Read the model definition and answer for the solid it produces. Units are mm, in the model's axes. A direction names the side the tool comes from. Coordinates: 2 decimals unless noted, no trailing zeros. Write each loop counter-clockwise with the first axis right and the second up, starting at its lowest first coordinate (ties: lowest second). Pieces come first, ordered by that corner, then holes.
(1) Which of the six approach directions +Z, -Z, +X, -X, +Y, -Y give full straight-line access (tool end or side, diameter ignored) to faces 4 (the cylindrical face through (-20.03, 6.31, 1.48)), 5 (the flat face through (-3, 14, 30)), 6 (the flat face through (-1, 16, 5))?
(2) Given pin 1 (21.5 mm diameter, centred on x = -9, y = -5, fed in from -Z); pin 2 (8 mm diameter, centred on y = 8, z = 17, fed in from +X); pin 3 (3 mm diameter, centred on x = 1, z = 19, fed in from -Y); pin 4 (12 mm diameter, centred on x = 14.5, z = 8.5, fed in from -Y), each flat-ended and moving along its own axis, determine where each tip first touches the part or whether it passes through.
(3) The part is cut by section A-A, the plane y = 0. Determine the outline of the cut face in (x, z).
(4) Straight lines are drawn through the part: line 1 along X through (y, z) = (0, 11); line 2 along Z through (x, y) = (16, 5.5). For each, find the intervals that lie inside material, in ascending order.
(5) Determine the mould class of faces 1 (the cylindrical face through (-12.932, -5.362, 14.79)), 2 (the cylindrical face through (4.769, -21.477, 3.992)), 3 (the flat face through (-4, 14, 0)) for opening direction Y: pulls with the +Y half, pulls with the -Y half, needs draft (parallel to the pull), parting line crosses it, or undercut.
(6) The part is cut by section C-C, the plane z = 7. Determine the outline of the cut face in (x, y).
Autodesk Inventor part; units mm, degrees
ref_plane "YZ Plane" through (0, 0, 0) normal (1, 0, 0) x (0, 1, 0)
ref_plane "XZ Plane" through (0, 0, 0) normal (0, 1, 0) x (-1, 0, 0)
ref_plane "XY Plane" through (0, 0, 0) normal (0, 0, 1) x (1, 0, 0)
sketch "Sketch1" plane through (0, 0, 0) normal (0, 1, 0) x (-1, 0, 0)
  line L0 (0, 0) -> (0, 30)
  line L1 (15.8, 30) -> (15.8, 5)
  line L2 (15.8, 5) -> (22, 5)
  line L3 (22, 5) -> (22, 3)
  line L4 (22, 3) -> (21, 3)
  line L5 (21, 3) -> (21, 0)
  line L6 (0, 30) -> (14, 30) construction
  line L7 (14, 30) -> (15.8, 30)
  line L8 (21, 0) -> (14, 0)
  line L9 (14, 0) -> (0, 0) construction
  line L10 (14, 30) -> (14, 0)
  dimension "d0" = 28
  dimension "d1" = 31.6
  dimension "d2" = 44
  dimension "d3" = 42
  dimension "d4" = 3
  dimension "d5" = 2
  dimension "d6" = 25
revolve "Revolution1" add sketch "Sketch1" angle 360 about axis through (0, 0, 0) along (0, 0, 1)
chamfer "Chamfer1" distance 0.4 angle 45 3 edges at (15.8, 0, 30) (22, 0, 5) (22, 0, 3)
properties part number "M42-nose-peace" material "Aluminum 6061"
Computed:
1. face 4: -Z
1. face 5: +Z, +X, -X, +Y, -Y
1. face 6: +Z
2. pin 1: stops at z = 0
2. pin 2: stops at x = 15.29
2. pin 3: stops at y = -15.8
2. pin 4: stops at y = -19.63
3. outline: (-22, 3.4) - (-21.6, 3) - (-21, 3) - (-21, 0) - (-14, 0) - (-14, 30) - (-15.4, 30) - (-15.8, 29.6) - (-15.8, 5) - (-21.6, 5) - (-22, 4.6) - close; (14, 0) - (21, 0) - (21, 3) - (21.6, 3) - (22, 3.4) - (22, 4.6) - (21.6, 5) - (15.8, 5) - (15.8, 29.6) - (15.4, 30) - (14, 30) - close
4. line 1: x = -15.8 to -14, 14 to 15.8
4. line 2: z = 0 to 5
5. face 1: undercut
5. face 2: parting line crosses it
5. face 3: needs draft
6. outline: circle Ø31.6 at (0, 0); hole circle Ø28 at (0, 0)
